from build123d import *

# Parameters (mm, degrees)
F0_R     = 3.96875
F1_DEPTH = 12.7
F2_R     = 3.175
F3_DEPTH = 3.175
F4_R     = 3.175
F5_DEPTH = 3.175
F6_SIZE  = 0.254


with BuildPart() as f1:
    # F0 (on Top) → F1 (new body)
    with BuildSketch(Plane.XY):
        Circle(F0_R)
    extrude(amount=F1_DEPTH)

    # F2 (on Top) → F3 (join)
    with BuildSketch(Plane.XY):
        Circle(F2_R)
    extrude(amount=-F3_DEPTH)

    # F4 (on face) → F5 (join)
    with BuildSketch(Plane.XY.offset(12.7)):
        Circle(F4_R)
    extrude(amount=F5_DEPTH)

    # F6
    f6_edges = [f1.edges().sort_by_distance(p)[0] for p in [
        (-3.175, 0, 15.875),
        (-3.96875, 0, 12.7),
        (-3.96875, 0, 0),
        (-3.175, 0, -3.175),
    ]]
    chamfer(f6_edges, length=F6_SIZE)


solid = f1.part
Could you check a few things on this model? Use its own coordinates, in mm. A direction names the side the tool comes from. Round coordinates to 2 decimals unless told otherwise and drop trailing zeros. Loops run counter-clockwise (first coordinate to the right, second up) from the corner with the lowest first, then second, coordinate; pieces in that order, holes last. Notation, with made-up numbers: (16.25, 30.25) -> (21.25, 30.25) arc R35 ccw to (21.25, 66.25) -> close; hole circle Ø10 at (66, 36.25). An arc over 180 degrees is marked (long way). Use CSV: the item, a comma, the result in double quotes.
(1) If I drill on probe 1 along Z at (x, y) = (-0.25, 3.25); probe 2 along Y at (x, z) = (2, 2); probe 3 along X at (y, z) = (1.25, 10), over which ranges is the centre line in solid material (lowest first)? Write a range as [from, to].
Return value:
probe 1,"z = [0, 12.7]"
probe 2,"y = [-3.43, 3.43]"
probe 3,"x = [-3.77, 3.77]"
(2) Suppose I cut it at C-C on z = 0.75. Write out the boundary of the cut face in (x, y), plus the area to 3 significant figures.
Return value:
outline,"circle Ø7.94 at (0, 0)"
area,"49.5 mm²"
(3) Suppose I cut it at A-A on x = 0. Write out the boundary of the cut face in (y, z) (3 decimals).
Return value:
outline,"(-3.969, 0.254) -> (-3.715, 0) -> (-3.175, 0) -> (-3.175, -2.921) -> (-2.921, -3.175) -> (2.921, -3.175) -> (3.175, -2.921) -> (3.175, 0) -> (3.715, 0) -> (3.969, 0.254) -> (3.969, 12.446) -> (3.715, 12.7) -> (3.175, 12.7) -> (3.175, 15.621) -> (2.921, 15.875) -> (-2.921, 15.875) -> (-3.175, 15.621) -> (-3.175, 12.7) -> (-3.715, 12.7) -> (-3.969, 12.446) -> close"
(4) Will this pin go through, and if not, where does the flat tip stop? pin 1 Ø2 at (y, z) = (-2.5, 9) entering from +X.
Return value:
pin 1,"stops at x = 3.67"
(5) If we mould it in two halves opening along Z, with no side actions, what happens to faces 3 (the flat face through (0, 0, 15.875)), 4 (the cylindrical face through (-0.69, -3.1, 14.14)), 5 (the flat face through (0, 0, -3.175))? For each: +Z half, -Z half, draft (parallel to the pull), parting line (faces both ways), or undercut.
Return value:
face 3,"+Z half"
face 4,"draft"
face 5,"-Z half"
(6) For faces 1 (the cylindrical face through (-0.69, -3.1, -1.44)), 2 (the cylindrical face through (-0.86, -3.874, 6.265)), which set-ups out of +Z, -Z, +X, -X, +Y, -Y let a thin tool reach every point of the face, with its end or its side?
Return value:
face 1,"-Z"
face 2,"+Z, -Z"
